```python
from build123d import *

# Parameters (mm, degrees)
SKETCH037_W     = 2.4
SKETCH037_H     = 30.4
PAD019_DEPTH    = 15
SKETCH038_W     = 15
SKETCH038_H     = 30
POCKET018_DEPTH = 4
SKETCH039_W     = 50
SKETCH039_H     = 15
POCKET019_DEPTH = 56
PAD022_DEPTH    = 15


with BuildPart() as part:
    # Sketch037 → Pad019 (new body, symmetric)
    with BuildSketch(Plane.YZ):
        with BuildLine():
            Line((0, 0), (22, 0))
            ThreePointArc((26.8296291314, -3.7059047745), (25.043807145, -1.0332332985), (22, 0))
            Line((26.8296291314, -3.7059047745), (40.3058913312, -54))
            Line((50.3058913312, -54), (40.3058913312, -54))
            Line((50.3058913312, -54), (35.4205328152, 1.5529142706))
            ThreePointArc((35.4205328152, 1.5529142706), (33.2775464315, 4.7601200417), (29.6249778574, 6))
            Line((29.6249778574, 6), (0, 6))
            Line((-21.7, -6.8), (0, 6))
            Line((-21.7, -6.8), (-21.7, -41.2))
            Line((-11.7, -41.2), (-21.7, -41.2))
            Line((0, 0), (-11.7, -41.2))
        make_face()
        with Locations((-18.5, -24)):
            Rectangle(SKETCH037_W, SKETCH037_H, mode=Mode.SUBTRACT)
    extrude(amount=PAD019_DEPTH, both=True)

    # Sketch038 (on Face10 of Pad019) → Pocket018 (cut)
    with BuildSketch(Plane(origin=(0, -21.7, 0), x_dir=(0, 0, -1), z_dir=(0, -1, 0))):
        with Locations((24, 0)):
            Rectangle(SKETCH038_W, SKETCH038_H)
    extrude(amount=-POCKET018_DEPTH, mode=Mode.SUBTRACT)

    # Sketch039 (on Face17 of Pocket018) → Pocket019 (cut)
    with BuildSketch(Plane(origin=(0, 0, 6), x_dir=(0, -1, 0), z_dir=(0, 0, 1))):
        with Locations((-25.3058913312, 0)):
            Rectangle(SKETCH039_W, SKETCH039_H)
    extrude(amount=-POCKET019_DEPTH, mode=Mode.SUBTRACT)

    # Sketch043 (on Face9 of Pocket019) → Pad022 (join)
    with BuildSketch(Plane(origin=(7.5, 0, 0), x_dir=(0, 1, 0), z_dir=(-1, 0, 0))):
        Polygon((34.5023642209, 32.3409419612), (31.7311897424, 22.7325814346), (41.2447676172, 20.1834259259), (43.8324912398, 29.8409419612), align=None)
        with BuildLine():
            Line((22, 0), (29.6249778574, -6))
            ThreePointArc((29.6249778574, -6), (33.2775464315, -4.7601200417), (35.4205328152, -1.5529142706))
            Line((26.9994594018, 5.0735233958), (35.4205328152, -1.5529142706))
            ThreePointArc((22, 0), (25.561433488, 1.4905568091), (26.9994594018, 5.0735233958))
        make_face()
    extrude(amount=PAD022_DEPTH)


with BuildPart() as part_1:
    # Body016 placement: moved
    add(part.part.moved(Location((-242, 0, 0))))


solid = part_1.part
```
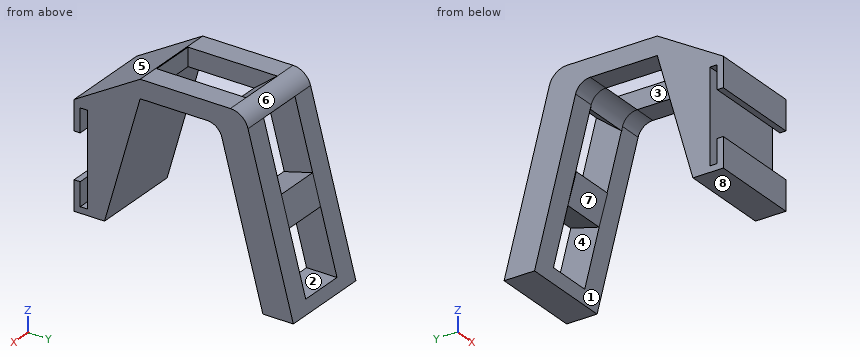
Could you check a few things on this model? Use its own coordinates, in mm. Face numbers are marked on the shaded views. A direction names the side the tool comes from. Round coordinates to 2 decimals unless told otherwise and drop trailing zeros. Write each loop counter-clockwise with the first axis right and the second up, starting at its lowest first coordinate (ties: lowest second). Pieces come first, ordered by that corner, then holes.
(1) Suppose I cut it at D-D on z = -8. Write out the boundary of the cut face in (x, y), and give its area (3 significant figures).
Findings below:
outline: (-257, -21.7) - (-227, -21.7) - (-227, -2.27) - (-257, -2.27) - close; (-257, 27.98) - (-249.5, 27.98) - (-249.5, 37.98) - (-257, 37.98) - close; (-234.5, 27.98) - (-227, 27.98) - (-227, 37.98) - (-234.5, 37.98) - close
area: 733 mm2
(2) Which directions (+Z, -Z, +X, -X, +Y, -Y) give clear straight access to the entire face, cutting with the end or side of a thin tool? Please do the marked faces 4, 5, 6, 7 and 8.
Findings below:
face 4: +Y
face 5: +Z, +X, -X, -Y
face 6: +Z, +X, -X, +Y
face 7: -Z, +X, -X
face 8: -Z, +X, -X, -Y
(3) Suppose I cut it at A-A on y = 17.5. Write out the boundary of the cut face in (x, z), and give its area (3 significant figures).
Findings below:
outline: (-257, 0) - (-249.5, 0) - (-249.5, 6) - (-257, 6) - close; (-234.5, 0) - (-227, 0) - (-227, 6) - (-234.5, 6) - close
area: 90.0 mm2
(4) Suppose I cut it at C-C on z = -29. Write out the boundary of the cut face in (x, y).
Findings below:
outline: (-257, -17.3) - (-227, -17.3) - (-227, -8.24) - (-257, -8.24) - close; (-257, 33.61) - (-249.5, 33.61) - (-249.5, 33.54) - (-234.5, 33.54) - (-234.5, 33.61) - (-227, 33.61) - (-227, 43.61) - (-257, 43.61) - close
(5) For pin 1 (2 mm diameter, centred on x = -245.5, z = 0, fed in from +Y); pin 2 (4 mm diameter, centred on x = -245, z = -30, fed in from +Y); pin 3 (10 mm diameter, centred on x = -251, z = -24.5, fed in from +Y), each with a flat end and sliding along its axis, tell me the tip position at first contact or that it passes through.
Findings below:
pin 1: stops at y = 34.72
pin 2: stops at y = 43.83
pin 3: stops at y = 43.74
(6) Thinking about a two-plate mould opening in Z: for the marked faces 1, 2 and 3, which applies, +Z half, -Z half, draft (parallel to the pull), parting line (faces both ways), or undercut?
Findings below:
face 1: -Z half
face 2: undercut
face 3: draft
(7) If I drill on probe 1 along X at (y, z) = (20, 2); probe 2 along Y at (x, z) = (-250, -12.5); probe 3 along Y at (x, z) = (-250, -22), over which ranges is the centre line in solid material (lowest first)?
Findings below:
probe 1: x = -257 to -249.5, -234.5 to -227
probe 2: y = -21.7 to -19.7, -17.3 to -3.55, 29.19 to 39.19
probe 3: y = -17.3 to -6.25, 31.73 to 41.73
(8) Suppose I cut it at B-B on x = -236.25. Write out the boundary of the cut face in (y, z), and give its area (3 significant figures).
Findings below:
outline: (-21.7, -41.2) - (-11.7, -41.2) - (0, 0) - (0.31, 0) - (0.31, 6) - (0, 6) - (-21.7, -6.8) - (-21.7, -16.5) - (-19.7, -16.5) - (-19.7, -8.8) - (-17.3, -8.8) - (-17.3, -39.2) - (-19.7, -39.2) - (-19.7, -31.5) - (-21.7, -31.5) - close; (22, 0) arc R5 cw to (27, -5.07) - (35.42, 1.55) arc R6 ccw to (29.62, 6) - close; (31.73, -22.73) - (34.5, -32.34) - (43.83, -29.84) - (41.24, -20.18) - close; (39.23, -50) - (40.31, -54) - (50.31, -54) - (49.23, -50) - close
area: 752 mm2
